```python
from build123d import *

# Parameters (mm, degrees)
BASEFRAMESKETCH_W           = 15.8
BASEFRAMESKETCH_H           = 3.2
BASEFRAME_DEPTH             = 7.9
STUDSSKETCH_R               = 2.197938665
STUDS_DEPTH                 = 1.6
MAINSTUDSPATTERN_COUNT      = 2
MAINSTUDSPATTERN_PITCH      = 8
MAINSTUDSPATTERN_COUNT_DIR2 = 2
MAINSTUDSPATTERN_PITCH_DIR2 = 8
MAINBASESHELL_T             = -1.2
UNDERCIRCLESKETCH_R         = 3.25
UNDERCIRCLESKETCH_R_2       = 2.4
UNDERCIRCLEEXTRUDE_DEPTH    = 1.8
ASHAPEDEDGECUT_DEPTH        = 2
FILLET13_R                  = 1


with BuildPart() as part:
    # BaseFrameSketch → BaseFrame (new, symmetric)
    with BuildSketch(Plane.XY):
        with Locations((-4.584729064, 1.6)):
            Rectangle(BASEFRAMESKETCH_W, BASEFRAMESKETCH_H)
    extrude(amount=BASEFRAME_DEPTH, both=True)

    # StudsSketch → Studs (add)
    with BuildSketch(Plane(origin=(0, 3.2, 0), x_dir=(1, 0, 0), z_dir=(0, 1, 0))):
        with Locations((-8.584729064, 4)):
            Circle(STUDSSKETCH_R)
    studs = extrude(amount=STUDS_DEPTH)

    # MainStudsPattern: Studs 2 × 2
    with Locations(*[(i * MAINSTUDSPATTERN_PITCH, 0, j * MAINSTUDSPATTERN_PITCH_DIR2) for i in range(MAINSTUDSPATTERN_COUNT) for j in range(MAINSTUDSPATTERN_COUNT_DIR2) if (i, j) != (0, 0)]):
        add(studs)

    # MainBaseShell
    mainbaseshell_openings = [part.faces().sort_by_distance(p)[0] for p in [
        (-4.584729064, 0, 0),
    ]]
    offset(amount=MAINBASESHELL_T, openings=mainbaseshell_openings, kind=Kind.INTERSECTION)

    # UnderCircleSketch → UnderCircleExtrude (add)
    with BuildSketch(Plane(origin=(0, 2, 0), x_dir=(-1, 0, 0), z_dir=(0, -1, 0))):
        with Locations(Location((4.584729064, 0, 0), (0, 0, 270))):
            Circle(UNDERCIRCLESKETCH_R)
        with Locations(Location((4.584729064, 0, 0), (0, 0, 270))):
            Circle(UNDERCIRCLESKETCH_R_2, mode=Mode.SUBTRACT)
    extrude(amount=UNDERCIRCLEEXTRUDE_DEPTH)

    # Sweep1: sweep along a curve in space
    with BuildLine() as sweep1_path:
        Line((3.315270936, 0, 7.9), (3.315270936, 3.2, 7.9))
    # Sketch10 → Sweep1 (sweep)
    with BuildSketch(Plane(origin=(0, 3.2, 0), x_dir=(1, 0, 0), z_dir=(0, 1, 0))):
        Polygon((-12.484729064, 7.9), (-20.484729064, -15.9), (-12.484729064, -15.9), align=None)
        Polygon((3.315270936, 7.9), (3.315270936, -15.9), (11.315270936, -15.9), align=None)
    sweep(path=sweep1_path.line)

    # Sketch11 → AShapedEdgeCut (cut)
    with BuildSketch(Plane(origin=(0, 0, 0), x_dir=(-1, 0, 0), z_dir=(0, -1, 0))):
        Polygon((-3.315270936, 3.352483875), (-3.598074089, 3.352483875), (-5.380624164, -1.900141374), (-6.136343318, -1.900141374), (-7.584500421, -6.930903588), (-3.315270936, -6.930903588), (-3.315270936, -4.81), (-5.328079185, -4.81), (-5.328079185, -3.61), (-3.315270936, -3.61), align=None)
        Polygon((-7.759680606, -8.895572671), (-7.759680606, -9.725211817), (-6.559680606, -9.725211817), (-6.559680606, -8.130903588), (-4.406736771, -8.130903588), (-4.406736771, -14.91), (-9.466166686, -14.91), (-9.466166686, -14.321814496), (-9.687501352, -14.236531964), (-8.150050802, -8.895572671), align=None)
        Polygon((-2.115270936, 4.601321399), (-2.895270936, 4.601321399), (-2.295270936, 6.7), (-2.115270936, 6.7), align=None)
        Polygon((11.284729064, 4.601321399), (11.284729064, 6.7), (11.464729064, 6.7), (12.064729064, 4.601321399), align=None)
        Polygon((13.576194899, -14.91), (18.635624814, -14.91), (18.635624814, -14.321814496), (18.85695948, -14.236531964), (17.31950893, -8.895572671), (16.929138734, -8.895572671), (16.929138734, -9.725211817), (15.729138734, -9.725211817), (15.729138734, -8.130903588), (13.576194899, -8.130903588), align=None)
        Polygon((12.484729064, -4.81), (12.484729064, -6.930903588), (16.753958549, -6.930903588), (15.305801446, -1.900141374), (14.550082292, -1.900141374), (12.767532217, 3.352483875), (12.484729064, 3.352483875), (12.484729064, -3.61), (14.497537313, -3.61), (14.497537313, -4.81), align=None)
    extrude(amount=-ASHAPEDEDGECUT_DEPTH, mode=Mode.SUBTRACT)

    # Fillet13
    fillet13_edges = [part.edges().sort_by_distance(p)[0] for p in [
        (3.315270936, 1.6, 7.9),
        (-12.484729064, 1.6, 7.9),
    ]]
    fillet(fillet13_edges, radius=FILLET13_R)


solid = part.part
```
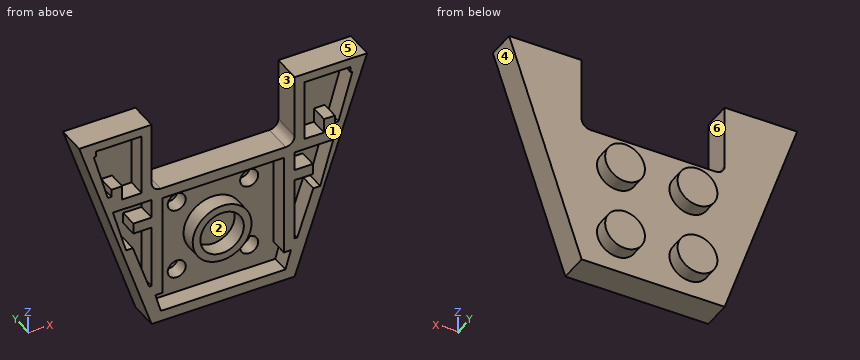
Verification items for the finished model (mm, model axes). Face numbers are marked on the shaded views. A direction names the side the tool comes from. Round coordinates to 2 decimals unless told otherwise and drop trailing zeros. Write each loop counter-clockwise with the first axis right and the second up, starting at its lowest first coordinate (ties: lowest second). Pieces come first, ordered by that corner, then holes.
1. Scan lines: L1, parallel to X at y = 1.5, z = 0; L2, parallel to Z at x = -3.5, y = 1.85; L3, parallel to Z at x = 1, y = 1.9. Record each from-to range of solid material in increasing order.
2. Section check B-B on y = 4.1. Enter the section's corners in (x, z).
3. Section check A-A on y = 2.35. Enter the section's corners in (x, z).
4. Gauge pin test, flat ends, axial feed: P1, Ø2.5, axis at x = -0.58, z = -4, coming from the -Y side; P2, Ø2, axis at y = 3.5, z = 1.5, coming from the -X side; P3, Ø0.6, axis at y = 1.5, z = 4.5, coming from the -X side. Record the tip position at first contact, or that the pin passes through.
5. Access from +Z, -Z, +X, -X, +Y, -Y to the whole of each face (thin tool, end or side, straight path). Record for the marked faces 1, 2 and 3.
6. Section check D-D on x = -4. Enter the section's corners in (y, z), plus the area to 3 significant figures.
7. Section check C-C on z = -5.75. Enter the section's corners in (x, y).
8. Draft check along X on the marked faces 4, 5 and 6. Enter one of: +X half, -X half, draft (parallel to the pull), parting line (faces both ways), or undercut.
Answer:
1. L1: x = -15.14 to -13.91, -12.48 to -11.28, -7.83 to -6.98, -2.18 to -1.33, 2.12 to 3.32, 4.74 to 5.97
1. L2: z = -7.9 to -6.7, -3.06 to -2.14, 2.14 to 3.06, 6.7 to 7.9
1. L3: z = -7.9 to -6.7, 6.7 to 7.9
2. outline: circle Ø4.4 at (-8.58, -4); circle Ø4.4 at (-8.58, 4); circle Ø4.4 at (-0.58, -4); circle Ø4.4 at (-0.58, 4)
3. outline: (-20.48, 15.9) - (-12.48, -7.9) - (3.32, -7.9) - (11.32, 15.9) - (3.32, 15.9) - (3.32, 8.9) arc R1 cw to (2.32, 7.9) - (-11.48, 7.9) arc R1 cw to (-12.48, 8.9) - (-12.48, 15.9) - close; hole circle Ø2 at (-8.58, -4); hole circle Ø2 at (-8.58, 4); hole circle Ø2 at (-0.58, -4); hole circle Ø2 at (-0.58, 4)
4. P1: stops at y = 2
4. P2: stops at x = -15.97
4. P3: stops at x = -16.75
5. face 1: +Z, -Z, +X, -X, -Y
5. face 2: -Y
5. face 3: +Z, +Y, -Y
6. outline: (0, -7.9) - (3.2, -7.9) - (3.2, 7.9) - (0, 7.9) - (0, 6.7) - (2, 6.7) - (2, 3.2) - (0.2, 3.2) - (0.2, 2.33) - (2, 2.33) - (2, -2.33) - (0.2, -2.33) - (0.2, -3.2) - (2, -3.2) - (2, -6.7) - (0, -6.7) - close
6. area: 26.9 mm2
7. outline: (-13.21, 0) - (-11.74, 0) - (-11.74, 2) - (2.57, 2) - (2.57, 0) - (4.04, 0) - (4.04, 3.2) - (0.75, 3.2) - (0.75, 4.8) - (-1.91, 4.8) - (-1.91, 3.2) - (-7.25, 3.2) - (-7.25, 4.8) - (-9.91, 4.8) - (-9.91, 3.2) - (-13.21, 3.2) - close
8. face 4: +X half
8. face 5: draft
8. face 6: undercut
